from build123d import *

# Parameters (mm, degrees)
SKETCH1_R           = 0.5
SKETCH1_R_2         = 4
SKETCH1_W           = 12
SKETCH1_H           = 4
BOSS_EXTRUDE1_DEPTH = 3


with BuildPart() as part:
    # Sketch1 → Boss-Extrude1 (new body)
    with BuildSketch(Plane(origin=(0, 0, 0), x_dir=(1, 0, 0), z_dir=(0, 1, 0))):
        with BuildLine():
            add(Edge.make_bspline(
                [(22.5, -16.5625), (34.262295129, -13.118708317), (45, -6.25)],
                knots=[0.479061635, 0.479061635, 0.479061635, 1, 1, 1], degree=2))
            ThreePointArc((45, -6.25), (47.588834765, 0), (45, 6.25))
            add(Edge.make_bspline(
                [(22.5, 16.5625), (34.262295129, 13.118708317), (45, 6.25)],
                knots=[0.479061635, 0.479061635, 0.479061635, 1, 1, 1], degree=2))
            Line((22.5, 16.5625), (0, 20))
            ThreePointArc((0, 20), (-20, 0), (0, -20))
            Line((0, -20), (22.5, -16.5625))
        make_face()
        with Locations(Location((0, -16.15, 0), (0, 0, 270))):
            Circle(SKETCH1_R, mode=Mode.SUBTRACT)
        with Locations(Location((0, -13.15, 0), (0, 0, 270))):
            Circle(SKETCH1_R, mode=Mode.SUBTRACT)
        with Locations(Location((0, -10.15, 0), (0, 0, 270))):
            Circle(SKETCH1_R, mode=Mode.SUBTRACT)
        with Locations(Location((-16.15, 0, 0), (0, 0, 270))):
            Circle(SKETCH1_R, mode=Mode.SUBTRACT)
        with BuildLine():
            ThreePointArc((-13.65, 0), (-13.15, 0.5), (-12.65, 0))
            ThreePointArc((-12.65, 0), (-13.15, -0.5), (-13.65, 0))
        make_face(mode=Mode.SUBTRACT)
        with BuildLine():
            ThreePointArc((-10.65, 0), (-10.15, 0.5), (-9.65, 0))
            ThreePointArc((-9.65, 0), (-10.15, -0.5), (-10.65, 0))
        make_face(mode=Mode.SUBTRACT)
        with BuildLine():
            ThreePointArc((-7.65, 0), (-7.15, 0.5), (-6.65, 0))
            ThreePointArc((-6.65, 0), (-7.15, -0.5), (-7.65, 0))
        make_face(mode=Mode.SUBTRACT)
        with Locations(Location((0, -7.15, 0), (0, 0, 270))):
            Circle(SKETCH1_R, mode=Mode.SUBTRACT)
        with Locations(Location((0, 0, 0), (0, 0, 270))):
            Circle(SKETCH1_R_2, mode=Mode.SUBTRACT)
        with Locations(Location((7.15, 0, 0), (0, 0, 270))):
            Circle(SKETCH1_R, mode=Mode.SUBTRACT)
        with Locations(Location((10.15, 0, 0), (0, 0, 270))):
            Circle(SKETCH1_R, mode=Mode.SUBTRACT)
        with Locations(Location((13.15, 0, 0), (0, 0, 270))):
            Circle(SKETCH1_R, mode=Mode.SUBTRACT)
        with Locations(Location((16.15, 0, 0), (0, 0, 270))):
            Circle(SKETCH1_R, mode=Mode.SUBTRACT)
        with Locations(Location((0, 7.15, 0), (0, 0, 270))):
            Circle(SKETCH1_R, mode=Mode.SUBTRACT)
        with Locations(Location((0, 10.15, 0), (0, 0, 270))):
            Circle(SKETCH1_R, mode=Mode.SUBTRACT)
        with Locations(Location((0, 13.15, 0), (0, 0, 270))):
            Circle(SKETCH1_R, mode=Mode.SUBTRACT)
        with Locations(Location((0, 16.15, 0), (0, 0, 270))):
            Circle(SKETCH1_R, mode=Mode.SUBTRACT)
        with Locations((31.5, 0)):
            Rectangle(SKETCH1_W, SKETCH1_H, mode=Mode.SUBTRACT)
    extrude(amount=BOSS_EXTRUDE1_DEPTH)


solid = part.part
Build history of the part. All positions in model axes, mm. A direction names the side the tool comes from. Give positions to 0.01 mm unless a question says otherwise; leave off trailing zeros. Loops run counter-clockwise (first coordinate to the right, second up) from the corner with the lowest first, then second, coordinate; pieces in that order, holes last. Notation, with made-up numbers: (4, 77) - (24, 77) arc R3 cw to (24, 82) - close; hole circle Ø11 at (15.25, 70.25). An arc over 180 degrees is marked (long way). Write item = value, one per line. Start each with the question number.
1) Drop flat-ended pins along their axis: pin 1 Ø1.5 at (y, z) = (2, 1) entering from -X; pin 2 Ø6.5 at (x, z) = (0, 0) entering from +Y; pin 3 Ø1.5 at (x, y) = (32, 2) entering from +Z. Give the stop position or say it passes through.
2) Tool access for faces 1 (the flat face through (31, 1, 2)), 2 (the flat face through (6, 0, 0)): list every direction of +Z, -Z, +X, -X, +Y, -Y with a clear straight run to the whole face (end or side of a thin tool).
3) Band-saw the part on C-C on y = 1.75. Count the separate pieces of the cut face and the enclosed holes in it, plus the area to 3 significant figures.
4) Band-saw the part on D-D on x = 14.5. Give the cut face in (y, z).
5) Pull direction Z, two halves, no side cores. Call faces 3 (the flat face through (6, 3, 0)), 4 (the cylindrical face through (47.59, 1.48, 0.1)), 5 (the flat face through (31, 1, -2)): +Z half, -Z half, draft (parallel to the pull), parting line (faces both ways), or undercut.
6) Band-saw the part on B-B on z = -3. Give the cut face in (x, y), plus the area to 3 significant figures.
7) Probe probe 1 along X at (y, z) = (0.5, -1); probe 2 along Z at (x, y) = (-3, 1.2); probe 3 along Z at (x, y) = (36, 1.55). List the from-to ranges inside material, lowest first. Write a range as from..to.
8) Band-saw the part on A-A on x = 2. Give the cut face in (y, z), plus the area to 3 significant figures.
Final values:
q1.pin_1 = -20
q1.pin_2 = through
q1.pin_3 = 13.47
q2.face_1 = +Y, -Y
q2.face_2 = +Z, -Z, +X, -X, -Y
q3.separate_pieces = 1
q3.enclosed_holes = 18
q3.area = 1,900 mm²
q4.outline = (0, -17.78) - (3, -17.78) - (3, 17.78) - (0, 17.78) - close
q5.face_3 = draft
q5.face_4 = parting line
q5.face_5 = undercut
q6.outline = (-19.77, 0) - (-2.65, 0) - (-2.65, 3) - (-19.77, 3) - close; (2.65, 0) - (47.06, 0) - (47.06, 3) - (2.65, 3) - close
q6.area = 185 mm²
q7.probe_1 = -19.97..-3.87, 3.87..25.5, 37.5..47.53
q7.probe_2 = -19.77..-2.65, 2.65..19.77
q7.probe_3 = -11.32..-2, 2..11.32
q8.outline = (0, -19.69) - (3, -19.69) - (3, -3.46) - (0, -3.46) - close; (0, 3.46) - (3, 3.46) - (3, 19.69) - (0, 19.69) - close
q8.area = 97.4 mm²
